```python
from build123d import *

# Parameters (mm, degrees)
SKETCH_1_W          = 80
SKETCH_1_H          = 80
EXTRUDE_1_DEPTH     = 10
SKETCH_2_R          = 20
CUT_EXTRUDE_1_DEPTH = 5
SKETCH_3_R          = 2.5
CUT_EXTRUDE_2_DEPTH = 5


with BuildPart() as part:
    # Эскиз1 → Бобышка-Вытянуть1 (new body)
    with BuildSketch(Plane.XY):
        with Locations((40, 40)):
            Rectangle(SKETCH_1_W, SKETCH_1_H)
    extrude(amount=EXTRUDE_1_DEPTH)

    # Эскиз2 → Вырез-Вытянуть1 (cut)
    with BuildSketch(Plane.XY.offset(10)):
        with Locations((40, 40)):
            Circle(SKETCH_2_R)
    extrude(amount=-CUT_EXTRUDE_1_DEPTH, mode=Mode.SUBTRACT)

    # Эскиз3 → Вырез-Вытянуть2 (cut)
    with BuildSketch(Plane.XY.offset(5)):
        with Locations((32, 40)):
            Circle(SKETCH_3_R)
        with Locations((48, 40)):
            Circle(SKETCH_3_R)
    extrude(amount=-CUT_EXTRUDE_2_DEPTH, mode=Mode.SUBTRACT)


solid = part.part
```
For this review, take the finished solid that the model builds, in its own axes (mm). A direction names the side the tool comes from. Give positions to 0.01 mm unless a question says otherwise; leave off trailing zeros. Order: outer loops, then holes, each group sorted by start corner. A loop starts at its lowest first (then second) coordinate and runs counter-clockwise, first axis right, second up.
1) Wall thickness on line 1 (Y direction, x = 48, z = 3.65); line 2 (X direction, y = 47, z = 5.75) (3 decimals); line 3 (X direction, y = 34, z = 8.5): over which ranges is each line inside the solid? List them lowest first.
2) Take a section at A-A (y = 40). Give the boundary of the cut face in (x, z), then the cut area to 3 significant figures.
3) Take a section at C-C (z = 6.75). Give the boundary of the cut face in (x, y).
4) The part is to be moulded in two halves that separate along X. For faces 1 (the face through (30.6, 58.3, 10)), 2 (the face through (80, 39, 5)), 3 (the face through (31.46, 37.56, 2.54)), say which applies: released by +X, released by -X, zero draft, split by the parting line, or undercut.
5) Take a section at B-B (x = 40). Give the boundary of the cut face in (y, z).
6) Take a section at D-D (x = 48). Give the boundary of the cut face in (y, z).
7) For faces 4 (the face through (50.31, 39.04, 2.54)), 5 (the face through (59.076, 46.007, 7.535)), list the 3-axis set-ups (+Z, -Z, +X, -X, +Y, -Y) from which the entire face can be reached by the end or side of a thin tool; tool diameter is ignored.
8) Insertion check: pin 1 (2 mm diameter, centred on x = 20, z = 5.5, fed in from -Y); pin 2 (5 mm diameter, centred on x = 34, y = 41.5, fed in from +Z); pin 3 (4.5 mm diameter, centred on x = 48, y = 40, fed in from -Z). Each pin has a flat end and moves straight along its axis. Give the tip position at first contact, or say it passes through.
Derived:
1. line 1: y = 0 to 37.5, 42.5 to 80
1. line 2: x = 0 to 21.265, 58.735 to 80
1. line 3: x = 0 to 20.92, 59.08 to 80
2. outline: (0, 0) - (29.5, 0) - (29.5, 5) - (20, 5) - (20, 10) - (0, 10) - close; (34.5, 0) - (45.5, 0) - (45.5, 5) - (34.5, 5) - close; (50.5, 0) - (80, 0) - (80, 10) - (60, 10) - (60, 5) - (50.5, 5) - close
2. area: 550 mm2
3. outline: (0, 0) - (80, 0) - (80, 80) - (0, 80) - close; hole circle Ø40 at (40, 40)
4. face 1: zero draft
4. face 2: released by +X
4. face 3: undercut
5. outline: (0, 0) - (80, 0) - (80, 10) - (60, 10) - (60, 5) - (20, 5) - (20, 10) - (0, 10) - close
6. outline: (0, 0) - (37.5, 0) - (37.5, 5) - (21.67, 5) - (21.67, 10) - (0, 10) - close; (42.5, 0) - (80, 0) - (80, 10) - (58.33, 10) - (58.33, 5) - (42.5, 5) - close
7. face 4: +Z, -Z
7. face 5: +Z
8. pin 1: stops at y = 0
8. pin 2: stops at z = 5
8. pin 3: passes through
